from build123d import *

# Parameters (mm, degrees)
SKETCH1_W           = 124
SKETCH1_H           = 84
BOSS_EXTRUDE1_DEPTH = 10
CUT_EXTRUDE1_DEPTH  = 2
SKETCH3_W           = 120.6
SKETCH3_H           = 60.6
CUT_EXTRUDE2_DEPTH  = 5
SKETCH4_W           = 45
SKETCH4_H           = 10
CUT_EXTRUDE3_DEPTH  = 5
FILLET1_R           = 3
FILLET2_R           = 5
SKETCH5_R           = 1.6
CUT_EXTRUDE4_DEPTH  = 238.548265663
SKETCH7_W           = 5.6
SKETCH7_H           = 7
CUT_EXTRUDE5_DEPTH  = 4
SKETCH8_W           = 100.6
SKETCH8_H           = 2
SKETCH8_W_2         = 2
SKETCH8_H_2         = 60.6
BOSS_EXTRUDE2_DEPTH = 5
FILLET3_R           = 2


with BuildPart() as part:
    # Sketch1 → Boss-Extrude1 (new body)
    with BuildSketch(Plane(origin=(0, 0, 0), x_dir=(1, 0, 0), z_dir=(0, 1, 0))):
        with Locations((-159.312972905, -43.940366204)):
            Rectangle(SKETCH1_W, SKETCH1_H)
    extrude(amount=BOSS_EXTRUDE1_DEPTH)

    # Sketch2 → Cut-Extrude1 (cut)
    with BuildSketch(Plane(origin=(0, 10, 0), x_dir=(1, 0, 0), z_dir=(0, 1, 0))):
        Polygon((-214.663225437, -3.640366204), (-219.612972905, -8.590113673), (-219.612972905, -79.590113673), (-214.962720373, -84.240366204), (-103.962720373, -84.240366204), (-99.012972905, -79.290618736), (-99.012972905, -8.290618736), (-103.663225437, -3.640366204), align=None)
    extrude(amount=-CUT_EXTRUDE1_DEPTH, mode=Mode.SUBTRACT)

    # Sketch3 → Cut-Extrude2 (cut)
    with BuildSketch(Plane(origin=(0, 8, 0), x_dir=(1, 0, 0), z_dir=(0, 1, 0))):
        with Locations((-159.312972905, -43.940366204)):
            Rectangle(SKETCH3_W, SKETCH3_H)
    extrude(amount=-CUT_EXTRUDE2_DEPTH, mode=Mode.SUBTRACT)

    # Sketch4 → Cut-Extrude3 (cut)
    with BuildSketch(Plane(origin=(0, 8, 0), x_dir=(1, 0, 0), z_dir=(0, 1, 0))):
        with Locations((-187.112972905, -8.640366204)):
            Rectangle(SKETCH4_W, SKETCH4_H)
        with Locations((-131.512972905, -8.640366204)):
            Rectangle(SKETCH4_W, SKETCH4_H)
        with Locations((-131.512972905, -79.240366204)):
            Rectangle(SKETCH4_W, SKETCH4_H)
        with Locations((-187.112972905, -79.240366204)):
            Rectangle(SKETCH4_W, SKETCH4_H)
    extrude(amount=-CUT_EXTRUDE3_DEPTH, mode=Mode.SUBTRACT)

    # Fillet1
    fillet1_edges = [part.edges().sort_by_distance(p)[0] for p in [
        (-209.612972905, 5.5, 74.240366204),
        (-164.612972905, 5.5, 74.240366204),
        (-109.012972905, 5.5, 74.240366204),
        (-154.012972905, 5.5, 74.240366204),
        (-154.012972905, 5.5, 13.640366204),
        (-109.012972905, 5.5, 13.640366204),
        (-209.612972905, 5.5, 13.640366204),
        (-164.612972905, 5.5, 13.640366204),
    ]]
    fillet(fillet1_edges, radius=FILLET1_R)

    # Fillet2
    fillet2_edges = [part.edges().sort_by_distance(p)[0] for p in [
        (-221.312972905, 5, 1.940366204),
        (-97.312972905, 5, 1.940366204),
        (-97.312972905, 5, 85.940366204),
        (-221.312972905, 5, 85.940366204),
    ]]
    fillet(fillet2_edges, radius=FILLET2_R)

    # Sketch5 → Cut-Extrude4 (cut, through all)
    with BuildSketch(Plane(origin=(0, 8, 0), x_dir=(1, 0, 0), z_dir=(0, 1, 0))):
        with Locations(Location((-214.312972905, -8.940366204, 0), (0, 0, 270))):
            Circle(SKETCH5_R)
        with Locations(Location((-159.312972905, -8.940366204, 0), (0, 0, 270))):
            Circle(SKETCH5_R)
        with Locations(Location((-104.312972905, -8.940366204, 0), (0, 0, 270))):
            Circle(SKETCH5_R)
        with Locations(Location((-104.312972905, -78.940366204, 0), (0, 0, 270))):
            Circle(SKETCH5_R)
        with Locations(Location((-159.312972905, -78.940366204, 0), (0, 0, 270))):
            Circle(SKETCH5_R)
        with Locations(Location((-214.312972905, -78.940366204, 0), (0, 0, 270))):
            Circle(SKETCH5_R)
    extrude(amount=-CUT_EXTRUDE4_DEPTH, mode=Mode.SUBTRACT)

    # Sketch7 → Cut-Extrude5 (cut)
    with BuildSketch(Plane.XZ):
        with Locations((-104.312972905, 8.940366204)):
            Rectangle(SKETCH7_W, SKETCH7_H)
        with Locations((-159.312972905, 8.940366204)):
            Rectangle(SKETCH7_W, SKETCH7_H)
        with Locations((-214.312972905, 8.940366204)):
            Rectangle(SKETCH7_W, SKETCH7_H)
        with Locations((-214.312972905, 78.940366204)):
            Rectangle(SKETCH7_W, SKETCH7_H)
        with Locations((-159.312972905, 78.940366204)):
            Rectangle(SKETCH7_W, SKETCH7_H)
        with Locations((-104.312972905, 78.940366204)):
            Rectangle(SKETCH7_W, SKETCH7_H)
    extrude(amount=-CUT_EXTRUDE5_DEPTH, mode=Mode.SUBTRACT)

    # Sketch8 → Boss-Extrude2 (add)
    with BuildSketch(Plane(origin=(0, 8, 0), x_dir=(1, 0, 0), z_dir=(0, 1, 0))):
        with Locations((-159.312972905, -83.240366204)):
            Rectangle(SKETCH8_W, SKETCH8_H)
        with Locations((-218.612972905, -43.940366204)):
            Rectangle(SKETCH8_W_2, SKETCH8_H_2)
        with Locations((-159.312972905, -4.640366204)):
            Rectangle(SKETCH8_W, SKETCH8_H)
        with Locations((-100.012972905, -43.940366204)):
            Rectangle(SKETCH8_W_2, SKETCH8_H_2)
    extrude(amount=-BOSS_EXTRUDE2_DEPTH)

    # Fillet3
    fillet3_edges = [part.edges().sort_by_distance(p)[0] for p in [
        (-209.612972905, 5.5, 82.240366204),
        (-109.012972905, 5.5, 82.240366204),
        (-154.012972905, 5.5, 82.240366204),
        (-164.612972905, 5.5, 82.240366204),
        (-217.612972905, 5.5, 13.640366204),
        (-217.612972905, 5.5, 74.240366204),
        (-109.012972905, 5.5, 5.640366204),
        (-209.612972905, 5.5, 5.640366204),
        (-164.612972905, 5.5, 5.640366204),
        (-154.012972905, 5.5, 5.640366204),
        (-101.012972905, 5.5, 74.240366204),
        (-101.012972905, 5.5, 13.640366204),
    ]]
    fillet(fillet3_edges, radius=FILLET3_R)


solid = part.part
Read the model definition and answer for the solid it produces. Units are mm, in the model's axes. A direction names the side the tool comes from. Round coordinates to 2 decimals unless told otherwise and drop trailing zeros. Write each loop counter-clockwise with the first axis right and the second up, starting at its lowest first coordinate (ties: lowest second). Pieces come first, ordered by that corner, then holes.
1. Which of the six approach directions +Z, -Z, +X, -X, +Y, -Y give full straight-line access (tool end or side, diameter ignored) to faces 4 (the face through (-210.515, 5.465, 12.785)), 5 (the face through (-104.926, 6.028, 80.418)), 6 (the face through (-211.513, 2, 9))?
2. The part is cut by section C-C, the plane y = 6.75. State how many separate pieces and enclosed holes the cut face has, then the cut area to 3 significant figures.
3. The part is cut by section B-B, the plane x = -146.5. Determine the outline of the cut face in (y, z).
4. Straight lines are drawn through the part: L1, parallel to X at y = 8.75, z = 9.5; L2, parallel to X at y = 4.75, z = 32; L3, parallel to X at y = 7, z = 11.5. For each, find the intervals that lie inside material, in ascending order.
5. The part is cut by section A-A, the plane z = 50.5. Determine the outline of the cut face in (x, y).
6. Given pin 1 Ø4 at (x, z) = (-199, 34.5) entering from +Y; pin 2 Ø3 at (x, z) = (-159.31, 8.94) entering from +Y, each flat-ended and moving along its own axis, determine where each tip first touches the part or whether it passes through.
7. Determine the mould class of faces 1 (the face through (-97.313, 5, 44)), 2 (the face through (-160, 4, 77)), 3 (the face through (-219.887, 5.07, 3.444)) for opening direction X: pulls with the +X half, pulls with the -X half, needs draft (parallel to the pull), parting line crosses it, or undercut.
Values:
1. face 4: +Y
1. face 5: +Y, -Y
1. face 6: -Y
2. separate pieces: 1
2. enclosed holes: 7
2. area: 1,840 mm2
3. outline: (0, 1.94) - (10, 1.94) - (10, 3.64) - (8, 3.64) - (8, 5.64) - (3, 5.64) - (3, 82.24) - (8, 82.24) - (8, 84.24) - (10, 84.24) - (10, 85.94) - (0, 85.94) - close
4. L1: x = -221.31 to -219.61, -99.01 to -97.31
4. L2: x = -221.31 to -217.61, -101.01 to -97.31
4. L3: x = -221.31 to -209.74, -164.49 to -154.14, -108.89 to -97.31
5. outline: (-221.31, 0) - (-97.31, 0) - (-97.31, 10) - (-99.01, 10) - (-99.01, 8) - (-101.01, 8) - (-101.01, 3) - (-217.61, 3) - (-217.61, 8) - (-219.61, 8) - (-219.61, 10) - (-221.31, 10) - close
6. pin 1: stops at y = 3
6. pin 2: passes through
7. face 1: pulls with the +X half
7. face 2: undercut
7. face 3: pulls with the -X half
